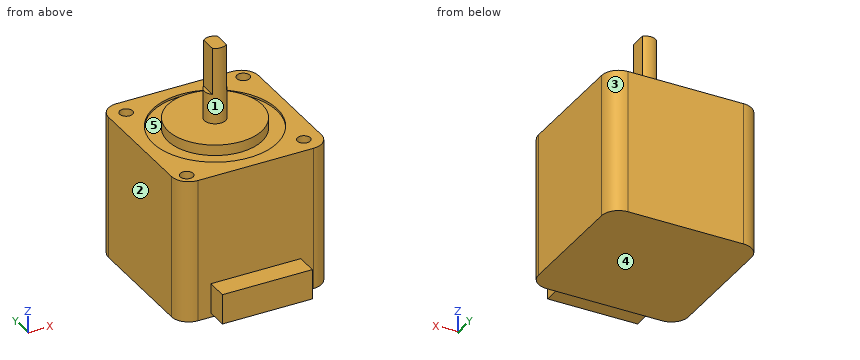
```python
from build123d import *

# Parameters (mm, degrees)
SKETCH1_W           = 35
SKETCH1_H           = 35
BOSS_EXTRUDE1_DEPTH = 33.5
SKETCH2_R           = 11
BOSS_EXTRUDE2_DEPTH = 2
CUT_EXTRUDE1_START  = -0.5
SKETCH3_R           = 14.5
SKETCH3_R_2         = 11
CUT_EXTRUDE1_DEPTH  = 0.5
FILLET1_R           = 4
SKETCH4_R           = 1.5
CUT_EXTRUDE2_DEPTH  = 5
SKETCH5_R           = 2.5
BOSS_EXTRUDE3_DEPTH = 18
CUT_EXTRUDE3_START  = -11
CUT_EXTRUDE3_DEPTH  = 11
SKETCH7_W           = 21
SKETCH7_H           = 7
BOSS_EXTRUDE4_DEPTH = 5


with BuildPart() as part:
    # Sketch1 → Boss-Extrude1 (new body)
    with BuildSketch(Plane.XY):
        Rectangle(SKETCH1_W, SKETCH1_H)
    extrude(amount=BOSS_EXTRUDE1_DEPTH)

    # Sketch2 → Boss-Extrude2 (add)
    with BuildSketch(Plane.XY.offset(33.5)):
        Circle(SKETCH2_R)
    extrude(amount=BOSS_EXTRUDE2_DEPTH)

    # Sketch3 → Cut-Extrude1 (cut)
    with BuildSketch(Plane.XY.offset(33.5).offset(CUT_EXTRUDE1_START)):
        Circle(SKETCH3_R)
        Circle(SKETCH3_R_2, mode=Mode.SUBTRACT)
    extrude(amount=CUT_EXTRUDE1_DEPTH, mode=Mode.SUBTRACT)

    # Fillet1
    fillet1_edges = [part.edges().sort_by_distance(p)[0] for p in [
        (17.5, -17.5, 16.75),
        (-17.5, -17.5, 16.75),
        (-17.5, 17.5, 16.75),
        (17.5, 17.5, 16.75),
    ]]
    fillet(fillet1_edges, radius=FILLET1_R)

    # Sketch4 → Cut-Extrude2 (cut)
    with BuildSketch(Plane.XY.offset(33.5)):
        with Locations((14.495689014, 14.495689014)):
            Circle(SKETCH4_R)
        with Locations((-14.495689014, -14.495689014)):
            Circle(SKETCH4_R)
        with Locations((-13.435028843, 13.435028843)):
            Circle(SKETCH4_R)
        with Locations((13.435028843, -13.435028843)):
            Circle(SKETCH4_R)
    extrude(amount=-CUT_EXTRUDE2_DEPTH, mode=Mode.SUBTRACT)

    # Sketch5 → Boss-Extrude3 (add)
    with BuildSketch(Plane.XY.offset(35.5)):
        Circle(SKETCH5_R)
    extrude(amount=BOSS_EXTRUDE3_DEPTH)

    # Sketch6 → Cut-Extrude3 (cut)
    with BuildSketch(Plane.XY.offset(53.5).offset(CUT_EXTRUDE3_START)):
        with BuildLine():
            Line((1.63546218, 1.890836708), (1.63546218, -1.890836708))
            ThreePointArc((1.63546218, -1.890836708), (2.5, 0), (1.63546218, 1.890836708))
        make_face()
        with BuildLine():
            Line((-1.63546218, 1.890836708), (-1.63546218, -1.890836708))
            ThreePointArc((-1.63546218, -1.890836708), (-2.5, 0), (-1.63546218, 1.890836708))
        make_face()
    extrude(amount=CUT_EXTRUDE3_DEPTH, mode=Mode.SUBTRACT)

    # Sketch7 → Boss-Extrude4 (add)
    with BuildSketch(Plane.XZ.offset(17.5)):
        with Locations((0, 4.5)):
            Rectangle(SKETCH7_W, SKETCH7_H)
    extrude(amount=BOSS_EXTRUDE4_DEPTH)


solid = part.part
```
The model under review builds one solid part; all positions refer to its coordinate system, in mm. Face numbers are marked on the shaded views. A direction names the side the tool comes from. Round coordinates to 2 decimals unless told otherwise and drop trailing zeros. Write each loop counter-clockwise with the first axis right and the second up, starting at its lowest first coordinate (ties: lowest second). Pieces come first, ordered by that corner, then holes. Notation, with made-up numbers: (8.5, -10) - (18.5, -10) arc R34 ccw to (18.5, 26) - close; hole circle Ø7 at (31.25, -1). An arc over 180 degrees is marked (long way). Answer as CSV lines item,"result". Start each with the question number.
(1) Draft analysis for pull direction X (two halves, no side actions). For the marked faces 3, 4 and 5, state which applies: pulls with the +X half, pulls with the -X half, needs draft (parallel to the pull), parting line crosses it, or undercut.
(2) We need section C-C on y = 0. State the section outline as (x, z) points, plus the area to 3 significant figures.
(3) We need section A-A on x = 0. State the section outline as (y, z) points, plus the area to 3 significant figures.
(4) For pin 1 Ø5 at (x, y) = (13.44, -13.44) entering from +Z; pin 2 Ø6 at (x, y) = (-2, -12.5) entering from -Z; pin 3 Ø2.5 at (x, y) = (-13.44, 13.44) entering from +Z; pin 4 Ø3 at (y, z) = (0, 48) entering from +X, all flat-tipped, find the tip position at first contact; note any pin that passes through.
(5) We need section D-D on x = -8.5. State the section outline as (y, z) points, plus the area to 3 significant figures.
(6) To check wall thickness, follow line 1 (Y direction, x = 0, z = 33.1); line 2 (X direction, y = -14, z = 32); line 3 (Z direction, x = -4, y = -11). State the ranges of each line that lie inside material, in increasing order.
(7) We need section B-B on z = 24. State the section outline as (x, y) points.
(8) For the marked faces 1 and 2, list the 3-axis set-ups (+Z, -Z, +X, -X, +Y, -Y) from which the entire face can be reached by the end or side of a thin tool; tool diameter is ignored.
Worked answers:
1,face 3,"pulls with the +X half"
1,face 4,"needs draft"
1,face 5,"undercut"
2,outline,"(-17.5, 0) - (17.5, 0) - (17.5, 33.5) - (14.5, 33.5) - (14.5, 33) - (11, 33) - (11, 35.5) - (2.5, 35.5) - (2.5, 42.5) - (1.64, 42.5) - (1.64, 53.5) - (-1.64, 53.5) - (-1.64, 42.5) - (-2.5, 42.5) - (-2.5, 35.5) - (-11, 35.5) - (-11, 33) - (-14.5, 33) - (-14.5, 33.5) - (-17.5, 33.5) - close"
2,area,"1,280 mm²"
3,outline,"(-22.5, 1) - (-17.5, 1) - (-17.5, 0) - (17.5, 0) - (17.5, 33.5) - (14.5, 33.5) - (14.5, 33) - (11, 33) - (11, 35.5) - (2.5, 35.5) - (2.5, 53.5) - (-2.5, 53.5) - (-2.5, 35.5) - (-11, 35.5) - (-11, 33) - (-14.5, 33) - (-14.5, 33.5) - (-17.5, 33.5) - (-17.5, 8) - (-22.5, 8) - close"
3,area,"1,340 mm²"
4,pin 1,"z = 33.5"
4,pin 2,"z = 0"
4,pin 3,"z = 28.5"
4,pin 4,"x = 1.64"
5,outline,"(-22.5, 1) - (-17.5, 1) - (-17.5, 0) - (17.5, 0) - (17.5, 33.5) - (11.75, 33.5) - (11.75, 33) - (6.98, 33) - (6.98, 35.5) - (-6.98, 35.5) - (-6.98, 33) - (-11.75, 33) - (-11.75, 33.5) - (-17.5, 33.5) - (-17.5, 8) - (-22.5, 8) - close"
5,area,"1,230 mm²"
6,line 1,"-17.5 to -14.5, -11 to 11, 14.5 to 17.5"
6,line 2,"-17.47 to -15.91, -13.08 to 12.05, 14.82 to 17.47"
6,line 3,"0 to 33"
7,outline,"(-17.5, -13.5) arc R4 ccw to (-13.5, -17.5) - (13.5, -17.5) arc R4 ccw to (17.5, -13.5) - (17.5, 13.5) arc R4 ccw to (13.5, 17.5) - (-13.5, 17.5) arc R4 ccw to (-17.5, 13.5) - close"
8,face 1,"+Z"
8,face 2,"+Z, -Z, -X, +Y, -Y"
